from build123d import *

# Parameters (mm, degrees)
EXTRUDE_1_DEPTH     = 35
SKETCH_2_R          = 28.5
EXTRUDE_2_DEPTH     = 69
EXTRUDE_START       = -9.5
EXTRUDE_3_DEPTH     = 9.5
SKETCH_4_R          = 24
EXTRUDE_4_DEPTH     = 3
SKETCH_5_R          = 7
EXTRUDE_5_DEPTH     = 31
SKETCH_6_R          = 2.75
CUT_EXTRUDE_1_DEPTH = 297
SKETCH_7_R          = 21
CUT_EXTRUDE_2_DEPTH = 22
EXTRUDE_6_DEPTH     = 17
CHAMFER_1_SIZE      = 0.5


with BuildPart() as part:
    # 草图1 → 凸台-拉伸1 (new body)
    with BuildSketch(Plane(origin=(0, 0, 0), x_dir=(1, 0, 0), z_dir=(0, 1, 0))):
        with BuildLine():
            Line((26.254761473, 28.5), (-26.254761473, 28.5))
            ThreePointArc((-26.254761473, 28.5), (-27.400387771, 27.400387771), (-28.5, 26.254761473))
            Line((-28.5, 26.254761473), (-28.5, -26.254761473))
            ThreePointArc((-28.5, -26.254761473), (-27.400387771, -27.400387771), (-26.254761473, -28.5))
            Line((-26.254761473, -28.5), (26.254761473, -28.5))
            ThreePointArc((26.254761473, -28.5), (27.400387771, -27.400387771), (28.5, -26.254761473))
            Line((28.5, -26.254761473), (28.5, 26.254761473))
            ThreePointArc((28.5, 26.254761473), (27.400387771, 27.400387771), (26.254761473, 28.5))
        make_face()
    extrude(amount=EXTRUDE_1_DEPTH)

    # 草图2 → 凸台-拉伸2 (add)
    with BuildSketch(Plane(origin=(0, 35, 0), x_dir=(1, 0, 0), z_dir=(0, 1, 0))):
        with Locations(Location((0, 0, 0), (0, 0, 270))):
            Circle(SKETCH_2_R)
    extrude(amount=EXTRUDE_2_DEPTH)

    # 草图3 → 凸台-拉伸3 (add)
    with BuildSketch(Plane(origin=(0, 104, 0), x_dir=(1, 0, 0), z_dir=(0, 1, 0)).offset(EXTRUDE_START)):
        with BuildLine():
            Line((-26.254761473, -28.5), (26.254761473, -28.5))
            ThreePointArc((26.254761473, -28.5), (27.400387771, -27.400387771), (28.5, -26.254761473))
            Line((28.5, -26.254761473), (28.5, 26.254761473))
            ThreePointArc((28.5, 26.254761473), (27.400387771, 27.400387771), (26.254761473, 28.5))
            Line((26.254761473, 28.5), (-26.254761473, 28.5))
            ThreePointArc((-26.254761473, 28.5), (-27.400387771, 27.400387771), (-28.5, 26.254761473))
            Line((-28.5, 26.254761473), (-28.5, -26.254761473))
            ThreePointArc((-28.5, -26.254761473), (-27.400387771, -27.400387771), (-26.254761473, -28.5))
        make_face()
    extrude(amount=EXTRUDE_3_DEPTH)

    # 草图4 → 凸台-拉伸4 (add)
    with BuildSketch(Plane(origin=(0, 104, 0), x_dir=(1, 0, 0), z_dir=(0, 1, 0))):
        with Locations(Location((0, 0, 0), (0, 0, 270))):
            Circle(SKETCH_4_R)
    extrude(amount=EXTRUDE_4_DEPTH)

    # 草图5 → 凸台-拉伸5 (add)
    with BuildSketch(Plane(origin=(0, 107, 0), x_dir=(1, 0, 0), z_dir=(0, 1, 0))):
        with Locations(Location((0, 0, 0), (0, 0, 270))):
            Circle(SKETCH_5_R)
    extrude(amount=EXTRUDE_5_DEPTH)

    # 草图6 → 切除-拉伸1 (cut)
    with BuildSketch(Plane.XZ):
        with Locations(Location((-23.582011153, 23.582011153, 0), (0, 0, 270))):
            Circle(SKETCH_6_R)
        with Locations(Location((23.582011153, 23.582011153, 0), (0, 0, 270))):
            Circle(SKETCH_6_R)
        with Locations(Location((23.582011153, -23.582011153, 0), (0, 0, 270))):
            Circle(SKETCH_6_R)
        with Locations(Location((-23.582011153, -23.582011153, 0), (0, 0, 270))):
            Circle(SKETCH_6_R)
    extrude(amount=-CUT_EXTRUDE_1_DEPTH, mode=Mode.SUBTRACT)

    # 草图7 → 切除-拉伸2 (cut)
    with BuildSketch(Plane.XZ):
        with Locations(Location((0, 0, 0), (0, 0, 270))):
            Circle(SKETCH_7_R)
    extrude(amount=-CUT_EXTRUDE_2_DEPTH, mode=Mode.SUBTRACT)

    # 草图8 → 凸台-拉伸6 (add)
    with BuildSketch(Plane.XZ.offset(-22)):
        with BuildLine():
            Line((-0.8, 3.919183588), (-0.8, 19.033194687))
            ThreePointArc((-0.8, 19.033194687), (-13.184507954, -13.750318178), (19.05, 0))
            ThreePointArc((19.05, 0), (13.750318178, 13.184507954), (0.8, 19.033194687))
            Line((0.8, 19.033194687), (0.8, 3.919183588))
            ThreePointArc((0.8, 3.919183588), (3.098386677, 2.529822128), (4, 0))
            ThreePointArc((4, 0), (-2.529822128, -3.098386677), (-0.8, 3.919183588))
        make_face()
    extrude(amount=EXTRUDE_6_DEPTH)

    # 倒角1
    chamfer_1_edges = [part.edges().sort_by_distance(p)[0] for p in [
        (0, 138, -7),
    ]]
    chamfer(chamfer_1_edges, length=CHAMFER_1_SIZE)


solid = part.part
The listing builds one solid part. Answer for the finished solid, in the listing's coordinates (mm). A direction names the side the tool comes from. Round coordinates to 2 decimals unless told otherwise and drop trailing zeros. Write each loop counter-clockwise with the first axis right and the second up, starting at its lowest first coordinate (ties: lowest second). Pieces come first, ordered by that corner, then holes. Notation, with made-up numbers: M 8.25,-18 L 19.25,-18 A23 ccw 19.25,13 Z; hole C -4.5,55.25 d2. An arc over 180 degrees is marked long. Write each question's results on one line, items separated by ' | '. Start each with the question number.
(1) Determine the mould class of faces 6 (the flat face through (-22, 94.5, -21)), 7 (the flat face through (-28.5, 17, 0)), 8 (the flat face through (4, 5, -4)) for opening direction Y: +Y half, -Y half, draft (parallel to the pull), parting line (faces both ways), or undercut.
(2) For faces 1 (the flat face through (-22, 94.5, 21)), 2 (the flat face through (22, 35, -21)), 3 (the flat face through (-22, 35, -21)), 4 (the cylindrical face through (-6.834, 122.036, -1.517)), 5 (the cylindrical face through (-27.82, 64.33, -6.18)), determine the directions among +Z, -Z, +X, -X, +Y, -Y from which every point of the face is accessible in a straight line to the end or side of a thin tool.
(3) The part is cut by section D-D, the plane x = 12.5. Write down the section's boundary in (y, z), and give its area (3 significant figures).
(4) Find the intervals of material crossed by line 1 (X direction, y = 12, z = 0); line 2 (Z direction, x = -24, y = 22); line 3 (X direction, y = 9, z = -11.5), in increasing order.
(5) The part is cut by section B-B, the plane x = -16. Write down the section's boundary in (y, z), and give its area (3 significant figures).
(6) The part is cut by section A-A, the plane z = 14.5. Write down the section's boundary in (x, y).
(7) The part is cut by section C-C, the plane y = 122. Write down the section's boundary in (x, z), and give its area (3 significant figures).
(8) Each of these flat-tipped pins is pushed along its axis until it touches: P1, Ø3, axis at x = 22, y = 86, coming from the -Z side; P2, Ø2, axis at x = 6, z = 9, coming from the +Y side; P3, Ø6.5, axis at x = -23.58, z = -23.58, coming from the -Y side; P4, Ø2, axis at x = -19.5, y = 48.5, coming from the -Z side. Where does it stop, or does it pass through?
Worked answers:
1) face 6: undercut | face 7: draft | face 8: -Y half
2) face 1: +Z, -X | face 2: -Z, +X | face 3: -Z, -X | face 4: +Y | face 5: none
3) outline: M 0,-28.5 L 35,-28.5 L 35,-25.61 L 94.5,-25.61 L 94.5,-28.5 L 104,-28.5 L 104,-20.49 L 107,-20.49 L 107,20.49 L 104,20.49 L 104,28.5 L 94.5,28.5 L 94.5,25.61 L 35,25.61 L 35,28.5 L 0,28.5 L 0,16.87 L 22,16.87 L 22,14.38 L 5,14.38 L 5,-14.38 L 22,-14.38 L 22,-16.87 L 0,-16.87 Z | area: 5,450 mm²
4) line 1: x = -28.5 to -21, -19.05 to -4, 4 to 19.05, 21 to 28.5 | line 2: z = -28.5 to -26.3, -20.86 to 20.86, 26.3 to 28.5 | line 3: x = -28.5 to -17.57, -15.19 to 15.19, 17.57 to 28.5
5) outline: M 0,-28.5 L 35,-28.5 L 35,-23.58 L 94.5,-23.58 L 94.5,-28.5 L 104,-28.5 L 104,-17.89 L 107,-17.89 L 107,17.89 L 104,17.89 L 104,28.5 L 94.5,28.5 L 94.5,23.58 L 35,23.58 L 35,28.5 L 0,28.5 L 0,13.6 L 22,13.6 L 22,10.34 L 5,10.34 L 5,-10.34 L 22,-10.34 L 22,-13.6 L 0,-13.6 Z | area: 5,200 mm²
6) outline: M -28.5,0 L -15.19,0 L -15.19,22 L -12.36,22 L -12.36,5 L -0.8,5 L -0.8,22 L 0.8,22 L 0.8,5 L 12.36,5 L 12.36,22 L 15.19,22 L 15.19,0 L 28.5,0 L 28.5,35 L 24.54,35 L 24.54,94.5 L 28.5,94.5 L 28.5,104 L 19.12,104 L 19.12,107 L -19.12,107 L -19.12,104 L -28.5,104 L -28.5,94.5 L -24.54,94.5 L -24.54,35 L -28.5,35 Z
7) outline: C 0,0 d14 | area: 154 mm²
8) P1: stops at z = -19.8 | P2: stops at y = 107 | P3: stops at y = 0 | P4: stops at z = -21.68
